Design review of the part built by this model. Coordinates are the model's own, in mm. Give positions to 0.01 mm unless a question says otherwise; leave off trailing zeros. Write each loop counter-clockwise with the first axis right and the second up, starting at its lowest first coordinate (ties: lowest second). Pieces come first, ordered by that corner, then holes.
```python
from build123d import *

# Parameters (mm, degrees)
SKETCH1_R           = 12.7
BOSS_EXTRUDE1_DEPTH = 5.08
SCALE1_SCALE        = 0.5


with BuildPart() as part:
    # Sketch1 → Boss-Extrude1 (new body)
    with BuildSketch(Plane.XY):
        with BuildLine():
            Line((93.467932513, -187.929219557), (-8.040338021, -204.583155787))
            ThreePointArc((-8.040338021, -204.583155787), (-88.944478372, -217.943504644), (-169.903751816, -204.921412232))
            Line((-169.903751816, -204.921412232), (-272.655005044, -188.283976468))
            ThreePointArc((-272.655005044, -188.283976468), (-300.456269849, -174.058121661), (-314.682124657, -146.256856856))
            Line((-314.682124657, -146.256856856), (-331.319560421, -43.505603627))
            ThreePointArc((-331.319560421, -43.505603627), (-344.341652832, 37.453669817), (-330.981303976, 118.357810167))
            Line((-330.981303976, 118.357810167), (-314.329829255, 219.851077431))
            ThreePointArc((-314.329829255, 219.851077431), (-300.11395964, 247.554656272), (-272.404769628, 261.75958564))
            Line((-272.404769628, 261.75958564), (-171.233737428, 278.317171496))
            ThreePointArc((-171.233737428, 278.317171496), (-89.808861292, 291.785970897), (-8.349194575, 278.529209999))
            Line((-8.349194575, 278.529209999), (93.484449571, 261.782540046))
            ThreePointArc((93.484449571, 261.782540046), (121.168832583, 247.570102588), (135.370852074, 219.880373742))
            Line((135.370852074, 219.880373742), (152.027133289, 118.357810167))
            ThreePointArc((152.027133289, 118.357810167), (165.388038657, 36.921062845), (152.027133289, -44.515684477))
            Line((152.027133289, -44.515684477), (135.373197059, -146.023955011))
            ThreePointArc((135.373197059, -146.023955011), (121.164420099, -173.720442597), (93.467932513, -187.929219557))
        make_face()
        with Locations((-89.477085343, 36.921062845)):
            Circle(SKETCH1_R, mode=Mode.SUBTRACT)
    extrude(amount=BOSS_EXTRUDE1_DEPTH)


with BuildPart() as part_1:
    # Scale1: scaled about (-89.546856293, 36.846362698, 2.54)
    add(part.part.scale(SCALE1_SCALE).moved(Location((-44.773428147, 18.423181349, 1.27))))


solid = part_1.part
```
(1) Consider section B-B, the plane z = 2.95. Give the boundary of the cut face in (x, y).
Resolved:
outline: (-210.43, -3.33) - (-202.11, -54.71) arc R25.4 ccw to (-181.1, -75.72) - (-129.73, -84.04) arc R127.43 ccw to (-48.79, -83.87) - (1.96, -75.54) arc R25.4 ccw to (22.91, -54.59) - (31.24, -3.83) arc R127.43 ccw to (31.24, 77.6) - (22.91, 128.36) arc R25.4 ccw to (1.97, 149.31) - (-48.95, 157.69) arc R127.43 ccw to (-130.39, 157.58) - (-180.98, 149.3) arc R25.4 ccw to (-201.94, 128.35) - (-210.26, 77.6) arc R127.43 ccw to start; hole circle Ø12.7 at (-89.51, 36.88)
(2) Mouldability with a two-part tool opening along Y and no side actions: class faces 1 (the face through (37.92, 37.46, 2.52)), 2 (the face through (-95.856, 37.163, 2.522)), 3 (the face through (-155.053, -79.936, 2.522)), 4 (the face through (15.654, 142.364, 2.522)) as pulls with the +Y half, pulls with the -Y half, needs draft (parallel to the pull), parting line crosses it, or undercut.
Resolved:
face 1: parting line crosses it
face 2: undercut
face 3: pulls with the -Y half
face 4: pulls with the +Y half
(3) Consider section C-C, the plane y = -21. Give the boundary of the cut face in (x, z), then the cut area to 3 significant figures.
Resolved:
outline: (-207.57, 1.27) - (28.42, 1.27) - (28.42, 3.81) - (-207.57, 3.81) - close
area: 599 mm2
(4) Clearance check with flat-ended pins moving along their axes: P1, Ø1, axis at x = 3.5, z = 3, coming from the -Y side; P2, Ø1.5, axis at y = 109, z = 3, coming from the +X side. State where each tip first meets the part, or that it passes through.
Resolved:
P1: stops at y = -75.35
P2: stops at x = 26.21
(5) Consider section D-D, the plane x = 13.5. Give the boundary of the cut face in (y, z).
Resolved:
outline: (-70.48, 1.27) - (144.25, 1.27) - (144.25, 3.81) - (-70.48, 3.81) - close
(6) Consider section A-A, the plane x = -91.5. Give the boundary of the cut face in (y, z).
Resolved:
outline: (-90.53, 1.27) - (30.85, 1.27) - (30.85, 3.81) - (-90.53, 3.81) - close; (42.91, 1.27) - (164.3, 1.27) - (164.3, 3.81) - (42.91, 3.81) - close
(7) To check wall thickness, follow L1, parallel to X at y = 34, z = 2.2; L2, parallel to Y at x = -88.5, z = 2.3; L3, parallel to X at y = 60, z = 2.2. State the ranges of each line that lie inside material, in increasing order.
Resolved:
L1: x = -216.91 to -95.17, -83.85 to 37.89
L2: y = -90.54 to 30.61, 43.15 to 164.31
L3: x = -214.83 to 35.81
